```python
from build123d import *

# Parameters (mm, degrees)
F0_W     = 0.7112
F0_H     = 12.7
F2_ANGLE = 340
F3_SIZE2 = 0.2286
F3_SIZE  = 0.3959468146


with BuildPart() as f2:
    # F0 (on Front) → F2 (revolve)
    with BuildSketch(Plane.XZ):
        with Locations((1.3081, -6.35)):
            Rectangle(F0_W, F0_H)
    revolve(axis=Axis((0, 0, -8.318349719), (0, 0, -1)), revolution_arc=F2_ANGLE)

    # F3
    f3_edges = [f2.edges().sort_by_distance(p)[0] for p in [
        (-1.638425, -0.288898, 0),
        (-1.638425, -0.288898, -12.7),
    ]]
    f3_side = f2.faces().sort_by_distance((-1.638425, -0.288898, -6.35))[0]
    chamfer(f3_edges, length=F3_SIZE, length2=F3_SIZE2, reference=f3_side)


solid = f2.part
```
Model file for the job. Use its own axes, mm. Coordinates: 2 decimals unless noted, no trailing zeros. Order: outer loops, then holes, each group sorted by start corner. A loop starts at its lowest first (then second) coordinate and runs counter-clockwise, first axis right, second up. Notation, with made-up numbers: M -8,-39 L 0,-39 A19 ccw 0,-29 Z; hole C 28,-33.5 d3. An arc over 180 degrees is marked long. Answer as CSV lines item,"result".
(1) Wall check: line 1 along Y through (x, z) = (0, -7.25); line 2 along X through (y, z) = (-0.55, -9.5); line 3 along Y through (x, z) = (-0.25, -7.5). Give the ranges that are in metal, low to high.
Geometry says:
line 1,"y = -1.66 to -0.95, 0.95 to 1.66"
line 2,"x = -1.57 to -0.78, 0.78 to 1.57"
line 3,"y = -1.64 to -0.92, 0.92 to 1.64"
(2) Pull direction Y, two halves, no side cores. Call faces 1 (the cylindrical face through (-0.93, -0.2, -6.26)), 2 (the cylindrical face through (-1.625, -0.357, -6.267)): +Y half, -Y half, draft (parallel to the pull), parting line (faces both ways), or undercut.
Geometry says:
face 1,"undercut"
face 2,"parting line"
(3) Band-saw the part on A-A, the plane x = 0. List the corners of the cut face in (y, z), then the cut area to 3 significant figures.
Geometry says:
outline,"M -1.66,-12.3 L -1.44,-12.7 L -0.95,-12.7 L -0.95,0 L -1.44,0 L -1.66,-0.4 Z; M 0.95,-12.7 L 1.44,-12.7 L 1.66,-12.3 L 1.66,-0.4 L 1.44,0 L 0.95,0 Z"
area,"17.9 mm2"
(4) Flat gauge pins, fed straight in: pin 1 (1 mm diameter, centred on y = -1, z = -11, fed in from +X); pin 2 (1.5 mm diameter, centred on x = -0.5, z = -2, fed in from +Y). Where does each tip first touch, or does it go through?
Geometry says:
pin 1,"stops at x = 1.59"
pin 2,"stops at y = 1.66"
